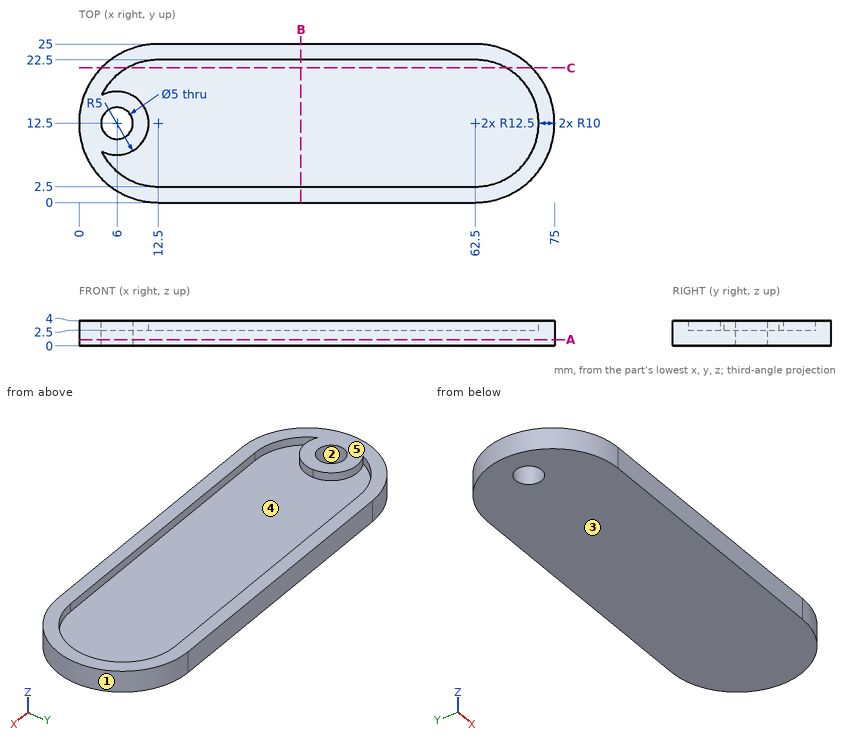
Check sheet for the drawn part. Datum: minimum x, y, z corner. Units: mm. A direction names the side the tool comes from. Give positions to 0.01 mm unless a question says otherwise; leave off trailing zeros. Write each loop counter-clockwise with the first axis right and the second up, starting at its lowest first coordinate (ties: lowest second). Pieces come first, ordered by that corner, then holes. Notation, with made-up numbers: (32, -29.5) -> (60, -29.5) arc R32 cw to (60, -3.5) -> close; hole circle Ø9 at (-2.75, 11). An arc over 180 degrees is marked (long way). Use one line per item in the form item = value. Start each with the question number.
1. Section check A-A (z = 1). Record the cut outline in (x, y).
2. Section check B-B (x = 35). Record the cut outline in (y, z).
3. Thickness scan on line 1 along X through (y, z) = (8, 2.95); line 2 along Y through (x, z) = (19.5, 3.1); line 3 along Y through (x, z) = (6, 3.2). Record the ranges inside material, lowest first. Write a range as from..to.
4. Section check C-C (y = 21.25). Record the cut outline in (x, z), and give its area (3 significant figures).
5. Access from +Z, -Z, +X, -X, +Y, -Y to the whole of each face (thin tool, end or side, straight path). Record for the marked faces 4 and 5.
6. Go/stop test with flat-tipped pins: P1, Ø3, axis at x = 6, y = 12.5, coming from the +Z side; P2, Ø1.5, axis at x = 12, y = 16, coming from the -Z side; P3, Ø6, axis at x = 48.5, y = 12, coming from the +Z side; P4, Ø1.5, axis at y = 5.5, z = 3, coming from the +X side. Record where each tip stops, or that it passes through.
7. Mould release check, pull along Y, two halves, no side actions. Record for the marked faces 1, 2 and 3: pulls with the +Y half, pulls with the -Y half, needs draft (parallel to the pull), parting line crosses it, or undercut.
Conclusion:
q1.outline = (12.5, 0) -> (62.5, 0) arc R12.5 ccw to (62.5, 25) -> (12.5, 25) arc R12.5 ccw to start; hole circle Ø5 at (6, 12.5)
q2.outline = (0, 0) -> (25, 0) -> (25, 4) -> (22.5, 4) -> (22.5, 2.5) -> (2.5, 2.5) -> (2.5, 4) -> (0, 4) -> close
q3.line_1 = 0.84..3.57, 3.82..8.18, 71.43..74.16
q3.line_2 = 0..2.5, 22.5..25
q3.line_3 = 1.82..4.9, 7.5..10, 15..17.5, 20.1..23.18
q4.outline = (3.57, 0) -> (71.43, 0) -> (71.43, 4) -> (67.34, 4) -> (67.34, 2.5) -> (7.66, 2.5) -> (7.66, 4) -> (3.57, 4) -> close
q4.area = 182 mm²
q5.face_4 = +Z
q5.face_5 = +Z, +X, -X, +Y, -Y
q6.P1 = through
q6.P2 = 0
q6.P3 = 2.5
q6.P4 = 73.33
q7.face_1 = parting line crosses it
q7.face_2 = undercut
q7.face_3 = needs draft
